from build123d import *

# Parameters (mm, degrees)
SKETCH1_W           = 5
SKETCH1_H           = 5
BOSS_EXTRUDE1_DEPTH = 1
SKETCH2_W           = 5
SKETCH2_H           = 1
BOSS_EXTRUDE2_DEPTH = 5
SKETCH3_W           = 5
SKETCH3_H           = 1
BOSS_EXTRUDE3_DEPTH = 1
SKETCH4_R           = 1
CUT_EXTRUDE1_DEPTH  = 1
SKETCH5_R           = 1
CUT_EXTRUDE2_DEPTH  = 1


with BuildPart() as part:
    # Sketch1 → Boss-Extrude1 (new body)
    with BuildSketch(Plane.XY):
        with Locations((-2.841614907, 1.055900621)):
            Rectangle(SKETCH1_W, SKETCH1_H)
    extrude(amount=BOSS_EXTRUDE1_DEPTH)

    # Sketch2 → Boss-Extrude2 (add)
    with BuildSketch(Plane.XY.offset(1)):
        with Locations((-2.841614907, 3.055900621)):
            Rectangle(SKETCH2_W, SKETCH2_H)
    extrude(amount=BOSS_EXTRUDE2_DEPTH)

    # Sketch3 → Boss-Extrude3 (add)
    with BuildSketch(Plane.XZ.offset(1.444099379)):
        with Locations((-2.841614907, 0.5)):
            Rectangle(SKETCH3_W, SKETCH3_H)
    extrude(amount=BOSS_EXTRUDE3_DEPTH)

    # Sketch4 → Cut-Extrude1 (cut)
    with BuildSketch(Plane.XY.offset(1)):
        with Locations((-2.841614907, 0.055900621)):
            Circle(SKETCH4_R)
    extrude(amount=-CUT_EXTRUDE1_DEPTH, mode=Mode.SUBTRACT)

    # Sketch5 → Cut-Extrude2 (cut)
    with BuildSketch(Plane.XZ.offset(-2.555900621)):
        with Locations((-2.841614907, 3.5)):
            Circle(SKETCH5_R)
    extrude(amount=-CUT_EXTRUDE2_DEPTH, mode=Mode.SUBTRACT)


solid = part.part
The listing builds one solid part. Answer for the finished solid, in the listing's coordinates (mm). A direction names the side the tool comes from. Coordinates: 2 decimals unless noted, no trailing zeros. Loops run counter-clockwise (first coordinate to the right, second up) from the corner with the lowest first, then second, coordinate; pieces in that order, holes last. Notation, with made-up numbers: (-5.75, 51) -> (2.25, 51) arc R20 cw to (2.25, 86) -> close; hole circle Ø9 at (81, 47.5). An arc over 180 degrees is marked (long way). Answer in a Markdown table with one row per item. Add a question column.
1. Determine the mould class of faces 3 (the flat face through (-5.342, 3, 2)), 4 (the cylindrical face through (-2.3, 3.05, 4.34)), 5 (the flat face through (-4, 2.556, 3)), 6 (the cylindrical face through (-2.38, -0.83, 0.51)) for opening direction X: +X half, -X half, draft (parallel to the pull), parting line (faces both ways), or undercut.
2. For faces 1 (the flat face through (-4, 0, 1)), 2 (the flat face through (-3, 3, 6)), determine the directions among +Z, -Z, +X, -X, +Y, -Y from which every point of the face is accessible in a straight line to the end or side of a thin tool.
3. The part is cut by section D-D, the plane x = -0.7. Write down the section's boundary in (y, z).
4. The part is cut by section B-B, the plane x = -2.6. Write down the section's boundary in (y, z).
5. The part is cut by section A-A, the plane z = 3.5. Write down the section's boundary in (x, y), then the cut area to 3 significant figures.
6. Flat-ended cylindrical pins translate along their axes: P1, Ø1.6, axis at x = -2.84, z = 3.5, coming from the +Y side; P2, Ø2.5, axis at x = -4, z = 4.5, coming from the -Y side; P3, Ø2, axis at x = -1, y = 1.5, coming from the -Z side; P4, Ø2.5, axis at x = -2.84, y = 0.06, coming from the +Z side. Find the tip coordinate at first contact, or state that the pin passes through.
7. The part is cut by section C-C, the plane y = 0.7. Write down the section's boundary in (x, z).
8. Consider line 1 (Y direction, x = -4.85, z = 3.05); line 2 (Z direction, x = -2.55, y = 1.5); line 3 (Y direction, x = -2.35, z = 0.5). Determine where each line is inside the solid, lowest interval first. Write a range as [from, to].
Answer below:
| question | item | result |
|---|---|---|
| 1 | face 3 | -X half |
| 1 | face 4 | undercut |
| 1 | face 5 | draft |
| 1 | face 6 | undercut |
| 2 | face 1 | +Z, +X, -X, -Y |
| 2 | face 2 | +Z, +X, -X, +Y, -Y |
| 3 | outline | (-2.44, 0) -> (3.56, 0) -> (3.56, 6) -> (2.56, 6) -> (2.56, 1) -> (-2.44, 1) -> close |
| 4 | outline | (-2.44, 0) -> (-0.91, 0) -> (-0.91, 1) -> (-2.44, 1) -> close; (1.03, 0) -> (3.56, 0) -> (3.56, 2.53) -> (2.56, 2.53) -> (2.56, 1) -> (1.03, 1) -> close; (2.56, 4.47) -> (3.56, 4.47) -> (3.56, 6) -> (2.56, 6) -> close |
| 5 | outline | (-5.34, 2.56) -> (-3.84, 2.56) -> (-3.84, 3.56) -> (-5.34, 3.56) -> close; (-1.84, 2.56) -> (-0.34, 2.56) -> (-0.34, 3.56) -> (-1.84, 3.56) -> close |
| 5 | area | 3.00 mm2 |
| 6 | P1 | through |
| 6 | P2 | y = 2.56 |
| 6 | P3 | z = 0 |
| 6 | P4 | z = 1 |
| 7 | outline | (-5.34, 0) -> (-3.61, 0) -> (-3.61, 1) -> (-5.34, 1) -> close; (-2.08, 0) -> (-0.34, 0) -> (-0.34, 1) -> (-2.08, 1) -> close |
| 8 | line 1 | [2.56, 3.56] |
| 8 | line 2 | [0, 1] |
| 8 | line 3 | [-2.44, -0.81], [0.93, 3.56] |
